```python
from build123d import *

# Parameters (mm, degrees)
BOSS_EXTRUDE1_DEPTH = 63.2
CUT_EXTRUDE14_REACH = 135.64
SKETCH31_R          = 19
CUT_EXTRUDE15_DEPTH = 60.2
CUT_EXTRUDE16_REACH = 135.64
SKETCH32_R          = 7
BOSS_EXTRUDE6_DEPTH = 2
FILLET1_R           = 10
SKETCH34_R          = 1.5
CUT_EXTRUDE17_DEPTH = 15


with BuildPart() as part:
    # Sketch1 → Boss-Extrude1 (new body)
    with BuildSketch(Plane(origin=(0, 0, 0), x_dir=(0, 0, -1), z_dir=(1, 0, 0))):
        with BuildLine():
            Line((0, 0), (114.8, 0))
            Line((114.8, 0), (114.8, 26.2))
            Line((114.8, 26.2), (109.8, 26.2))
            ThreePointArc((109.8, 26.2), (93.6, 10), (77.4, 26.2))
            Line((77.4, 26.2), (37.4, 26.2))
            ThreePointArc((37.4, 26.2), (21.2, 10), (5, 26.2))
            Line((5, 26.2), (0, 26.2))
            Line((0, 26.2), (0, 0))
        make_face()
    extrude(amount=BOSS_EXTRUDE1_DEPTH)

    # Sketch30 → Cut-Extrude14 (cut, up to next)
    with BuildSketch(Plane(origin=(0, 26.2, 0), x_dir=(1, 0, 0), z_dir=(0, 1, 0)), mode=Mode.PRIVATE) as cut_extrude14_sk1:
        Polygon((63.2, 75.375), (61.424647922, 76.4), (61.424647922, 71.1), (63.2, 72.125), align=None)
    cut_extrude14_tool1 = extrude(cut_extrude14_sk1.sketch, amount=-CUT_EXTRUDE14_REACH, mode=Mode.PRIVATE) & part.part
    # Sketch30 → Cut-Extrude14 (cut, up to next)
    with BuildSketch(Plane(origin=(0, 26.2, 0), x_dir=(1, 0, 0), z_dir=(0, 1, 0)), mode=Mode.PRIVATE) as cut_extrude14_sk2:
        Polygon((63.2, 42.675), (61.424647922, 43.7), (61.424647922, 38.4), (63.2, 39.425), align=None)
    cut_extrude14_tool2 = extrude(cut_extrude14_sk2.sketch, amount=-CUT_EXTRUDE14_REACH, mode=Mode.PRIVATE) & part.part
    add(cut_extrude14_tool1.solids().sort_by_distance((62.241379, 26.2, -73.75))[0], mode=Mode.SUBTRACT)
    add(cut_extrude14_tool2.solids().sort_by_distance((62.241379, 26.2, -41.05))[0], mode=Mode.SUBTRACT)

    # Sketch31 → Cut-Extrude15 (cut)
    with BuildSketch(Plane.ZY):
        with Locations((-57.4, 26.2)):
            Circle(SKETCH31_R)
    extrude(amount=-CUT_EXTRUDE15_DEPTH, mode=Mode.SUBTRACT)

    # Sketch32 → Cut-Extrude16 (cut, up to next)
    with BuildSketch(Plane(origin=(63.2, 0, 0), x_dir=(0, 0, -1), z_dir=(1, 0, 0)), mode=Mode.PRIVATE) as cut_extrude16_sk1:
        with Locations((57.4, 26.2)):
            Circle(SKETCH32_R)
    cut_extrude16_tool1 = extrude(cut_extrude16_sk1.sketch, amount=-CUT_EXTRUDE16_REACH, mode=Mode.PRIVATE) & part.part
    add(cut_extrude16_tool1.solids().sort_by_distance((63.2, 26.2, -57.4))[0], mode=Mode.SUBTRACT)

    # Sketch33 → Boss-Extrude6 (add)
    with BuildSketch(Plane.ZY):
        with BuildLine():
            Line((-74.4, 26.2), (-76.4, 26.2))
            ThreePointArc((-76.4, 26.2), (-57.4, 7.2), (-38.4, 26.2))
            Line((-38.4, 26.2), (-40.4, 26.2))
            ThreePointArc((-40.4, 26.2), (-57.4, 9.2), (-74.4, 26.2))
        make_face()
    extrude(amount=-BOSS_EXTRUDE6_DEPTH)

    # Fillet1
    fillet1_edges = [part.edges().sort_by_distance(p)[0] for p in [
        (31.6, 0, -114.8),
        (31.6, 0, 0),
    ]]
    fillet(fillet1_edges, radius=FILLET1_R)

    # Sketch34 → Cut-Extrude17 (cut)
    with BuildSketch(Plane(origin=(0, 26.2, 0), x_dir=(1, 0, 0), z_dir=(0, 1, 0))):
        with Locations(Location((9.6, 112.3, 0), (0, 0, 270))):
            Circle(SKETCH34_R)
        with Locations(Location((31.6, 112.3, 0), (0, 0, 270))):
            Circle(SKETCH34_R)
        with Locations(Location((53.6, 112.3, 0), (0, 0, 270))):
            Circle(SKETCH34_R)
        with Locations(Location((53.6, 2.5, 0), (0, 0, 90))):
            Circle(SKETCH34_R)
        with Locations(Location((31.6, 2.5, 0), (0, 0, 90))):
            Circle(SKETCH34_R)
        with Locations(Location((9.6, 2.5, 0), (0, 0, 90))):
            Circle(SKETCH34_R)
    extrude(amount=-CUT_EXTRUDE17_DEPTH, mode=Mode.SUBTRACT)


solid = part.part
```
Geometry: final body of the model. Coordinates: model frame, mm. A direction names the side the tool comes from. Round coordinates to 2 decimals unless told otherwise and drop trailing zeros. Write each loop counter-clockwise with the first axis right and the second up, starting at its lowest first coordinate (ties: lowest second). Pieces come first, ordered by that corner, then holes.
Item 1: Mould query, pull axis X, two halves, no side actions, for faces 1 (the face through (0, 7, -58)), 2 (the face through (32.04, 2.85, -111.79)), 3 (the face through (10, 11.2, -112)). Classes: +X half, -X half, draft (parallel to the pull), parting line (faces both ways), or undercut.
Item 2: Material intervals for L1, parallel to X at y = 16.75, z = -2.5; L2, parallel to Z at x = 24, y = 12.75; L3, parallel to X at y = 19, z = -41, sorted ascending.
Item 3: Section query B-B (x = 53.6). Return loops of the section in (y, z).
Item 4: Pin query (flat end, axial travel): P1, Ø2.5, axis at x = 31.6, z = -2.5, coming from the -Y side; P2, Ø1.5, axis at x = 10, z = -112, coming from the +Y side; P3, Ø1.6, axis at y = 11.5, z = -73, coming from the +X side. Return the tip coordinate at first contact, or that it passes through.
Item 5: Set-up query: faces 4 (the face through (0.986, 9.204, -57.026)), 5 (the face through (55.087, 18.805, -112.495)), 6 (the face through (31.158, 10.004, -21.556)). Return all of +Z, -Z, +X, -X, +Y, -Y with unobstructed straight access to the full face (end or side cutting, diameter ignored); none if empty.
Item 6: Section query A-A (y = 12.75). Give the number of separate pieces and of enclosed holes in the cut face, plus the area to 3 significant figures.
Item 7: Section query C-C (z = -62). Return loops of the section in (x, y).
Completed:
1. face 1: -X half
1. face 2: draft
1. face 3: undercut
2. L1: x = 0 to 8.1, 11.1 to 30.1, 33.1 to 52.1, 55.1 to 63.2
2. L2: z = -114.8 to -102.63, -84.57 to -70.82, -43.98 to -30.23, -12.17 to 0
2. L3: x = 0 to 2, 60.2 to 61.42
3. outline: (0, -104.8) arc R10 ccw to (10, -114.8) - (26.2, -114.8) - (26.2, -113.8) - (11.2, -113.8) - (11.2, -110.8) - (26.2, -110.8) - (26.2, -109.8) arc R16.2 cw to (26.2, -77.4) - (26.2, -76.4) arc R19 cw to (26.2, -38.4) - (26.2, -37.4) arc R16.2 cw to (26.2, -5) - (26.2, -4) - (11.2, -4) - (11.2, -1) - (26.2, -1) - (26.2, 0) - (10, 0) arc R10 ccw to (0, -10) - close
4. P1: stops at y = 2.19
4. P2: stops at y = 11.2
4. P3: stops at x = 61.42
5. face 4: -X, +Y
5. face 5: +Y
5. face 6: +X, -X, +Y
6. separate pieces: 3
6. enclosed holes: 6
6. area: 3,310 mm2
7. outline: (0, 0) - (63.2, 0) - (63.2, 20.92) - (60.2, 20.92) - (60.2, 7.77) - (2, 7.77) - (2, 9.83) - (0, 9.83) - close
